Could you check a few things on this model? Use its own coordinates, in mm. A direction names the side the tool comes from. Coordinates: 2 decimals unless noted, no trailing zeros. Loops run counter-clockwise (first coordinate to the right, second up) from the corner with the lowest first, then second, coordinate; pieces in that order, holes last.
1) Imagine slicing it at B-B on y = -8.5. Please give me the cut outline in (x, z) (3 decimals).
2) Thinking about a two-plate mould opening in X: for faces 1 (the face through (19.05, 4, 0)), 2 (the face through (-9.525, 0, -7)), 3 (the face through (0, 19.05, 0)), 4 (the face through (6, -3.175, -7)), which applies, released by +X, released by -X, zero draft, split by the parting line, or undercut?
3) Imagine slicing it at D-D on z = 0. Please give me the cut outline in (x, y) (3 decimals), plus the area to 3 significant figures.
4) Imagine slicing it at C-C on x = 11.5. Please give me the cut outline in (y, z) (3 decimals), plus the area to 3 significant figures.
5) Will these pins go through, and if not, where does the flat tip stop? P1, Ø6, axis at y = -15, z = -3.5, coming from the -X side; P2, Ø4, axis at y = -5, z = -7, coming from the +X side.
6) Imagine slicing it at A-A on z = 7. Please give me the cut outline in (x, y) (3 decimals).
7) For faces 5 (the face through (-25.31, -3.1, 0.69)), 6 (the face through (0, 3.175, 7)), 7 (the face through (31.75, 0, 0)), 8 (the face through (-3.175, 6, -7)), which set-ups out of +Z, -Z, +X, -X, +Y, -Y let a thin tool reach every point of the face, with its end or its side?
8) If I drill on line 1 along X through (y, z) = (-5, -5.75) (3 decimals); line 2 along X through (y, z) = (-3, 5); line 3 along X through (y, z) = (-8.5, 7), over which ranges is the centre line in solid material (lowest first)?
```python
from build123d import *

# Parameters (mm, degrees)
SKETCH1_W           = 38.1
SKETCH1_H           = 38.1
BOSS_EXTRUDE1_DEPTH = 9.525
SKETCH2_W           = 25.4
SKETCH2_H           = 6.35
CUT_EXTRUDE1_DEPTH  = 5.08
CUT_EXTRUDE2_DEPTH  = 5.08
SKETCH4_R           = 3.175
BOSS_EXTRUDE2_DEPTH = 12.7


with BuildPart() as part:
    # Sketch1 → Boss-Extrude1 (new body, symmetric)
    with BuildSketch(Plane.XY):
        Rectangle(SKETCH1_W, SKETCH1_H)
    extrude(amount=BOSS_EXTRUDE1_DEPTH, both=True)

    # Sketch2 → Cut-Extrude1 (cut)
    with BuildSketch(Plane.XY.offset(9.525)):
        Rectangle(SKETCH2_W, SKETCH2_H)
    extrude(amount=-CUT_EXTRUDE1_DEPTH, mode=Mode.SUBTRACT)

    # Sketch3 → Cut-Extrude2 (cut)
    with BuildSketch(Plane(origin=(0, 0, -9.525), x_dir=(-1, 0, 0), z_dir=(0, 0, -1))):
        Polygon((3.175, 3.175), (9.525, 3.175), (9.525, -3.175), (3.175, -3.175), (3.175, -9.525), (-3.175, -9.525), (-3.175, -3.175), (-9.525, -3.175), (-9.525, 3.175), (-3.175, 3.175), (-3.175, 9.525), (3.175, 9.525), align=None)
    extrude(amount=-CUT_EXTRUDE2_DEPTH, mode=Mode.SUBTRACT)

    # Sketch4 → Boss-Extrude2 (add)
    with BuildSketch(Plane(origin=(19.05, 0, 0), x_dir=(0, 0, -1), z_dir=(1, 0, 0))):
        Circle(SKETCH4_R)
    boss_extrude2 = extrude(amount=BOSS_EXTRUDE2_DEPTH)

    # Mirror1: Boss-Extrude2 across plane
    add(boss_extrude2.mirror(Plane(origin=(0, 0, 0), x_dir=(0, 0, 1), z_dir=(1, 0, 0))))


solid = part.part
```
Filled in:
1. outline: (-19.05, -9.525) - (-3.175, -9.525) - (-3.175, -4.445) - (3.175, -4.445) - (3.175, -9.525) - (19.05, -9.525) - (19.05, 9.525) - (-19.05, 9.525) - close
2. face 1: released by +X
2. face 2: undercut
2. face 3: zero draft
2. face 4: undercut
3. outline: (-31.75, -3.175) - (-19.05, -3.175) - (-19.05, -19.05) - (19.05, -19.05) - (19.05, -3.175) - (31.75, -3.175) - (31.75, 3.175) - (19.05, 3.175) - (19.05, 19.05) - (-19.05, 19.05) - (-19.05, 3.175) - (-31.75, 3.175) - close
3. area: 1,610 mm2
4. outline: (-19.05, -9.525) - (19.05, -9.525) - (19.05, 9.525) - (3.175, 9.525) - (3.175, 4.445) - (-3.175, 4.445) - (-3.175, 9.525) - (-19.05, 9.525) - close
4. area: 694 mm2
5. P1: stops at x = -19.05
5. P2: stops at x = 19.05
6. outline: (-19.05, -19.05) - (19.05, -19.05) - (19.05, 19.05) - (-19.05, 19.05) - close; hole (-12.7, -3.175) - (12.7, -3.175) - (12.7, 3.175) - (-12.7, 3.175) - close
7. face 5: -X
7. face 6: +Z
7. face 7: +Z, -Z, +X, +Y, -Y
7. face 8: -Z
8. line 1: x = -19.05 to -3.175, 3.175 to 19.05
8. line 2: x = -19.05 to -12.7, 12.7 to 19.05
8. line 3: x = -19.05 to 19.05
